```python
from build123d import *

# Parameters (mm, degrees)
F0_W     = 50.8
F0_H     = 50.8
F1_DEPTH = 25.4
F2_W     = 50.8
F2_H     = 25.4
F3_DEPTH = 25.4
F4_W     = 50.8
F4_H     = 76.2
F5_DEPTH = 25.4
F6_W     = 50.8
F6_H     = 101.6
F7_DEPTH = 25.4
F8_W     = 50.8
F8_H     = 127
F9_DEPTH = 25.4


with BuildPart() as f1:
    # F0 (on Top) → F1 (new body)
    with BuildSketch(Plane.XY):
        with Locations((25.4, 25.4)):
            Rectangle(F0_W, F0_H)
    extrude(amount=F1_DEPTH)

    # F2 (on face) → F3 (join)
    with BuildSketch(Plane.XY.offset(25.4)):
        with Locations((25.4, 38.1)):
            Rectangle(F2_W, F2_H)
    extrude(amount=F3_DEPTH)

    # F4 (on face) → F5 (join)
    with BuildSketch(Plane(origin=(0, 50.8, 0), x_dir=(-1, 0, 0), z_dir=(0, 1, 0))):
        with Locations((-25.4, 38.1)):
            Rectangle(F4_W, F4_H)
    extrude(amount=F5_DEPTH)

    # F6 (on face) → F7 (join)
    with BuildSketch(Plane(origin=(0, 0, 0), x_dir=(1, 0, 0), z_dir=(0, 0, -1))):
        with Locations((25.4, -25.4)):
            Rectangle(F6_W, F6_H)
    extrude(amount=F7_DEPTH)

    # F8 (on face) → F9 (join)
    with BuildSketch(Plane(origin=(0, 0, -25.4), x_dir=(1, 0, 0), z_dir=(0, 0, -1))):
        with Locations((25.4, -12.7)):
            Rectangle(F8_W, F8_H)
    extrude(amount=F9_DEPTH)


solid = f1.part
```
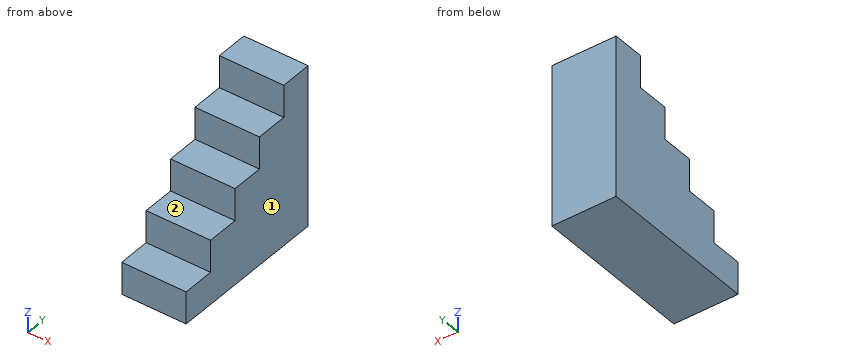
Verification items for the finished model (mm, model axes). Face numbers are marked on the shaded views. A direction names the side the tool comes from. Give positions to 0.01 mm unless a question says otherwise; leave off trailing zeros. Order: outer loops, then holes, each group sorted by start corner. A loop starts at its lowest first (then second) coordinate and runs counter-clockwise, first axis right, second up. Notation, with made-up numbers: M 55.5,62.25 L 84.5,62.25 A32 cw 84.5,96.25 Z; hole C 3,-28.75 d3. An arc over 180 degrees is marked long. Answer in a Markdown table with one row per item. Add a question column.
Item 1: Tool access check on the marked faces 1 and 2. Record the directions out of +Z, -Z, +X, -X, +Y, -Y that give a thin tool (end or side, any length) a straight path to the whole face; none if there is none.
Item 2: Gauge pin test, flat ends, axial feed: pin 1 (7.5 mm diameter, centred on x = 18, y = -13.5, fed in from +Z); pin 2 (12 mm diameter, centred on y = -27, z = -21, fed in from -X); pin 3 (7.5 mm diameter, centred on x = 18, z = 68.5, fed in from -Y); pin 4 (12 mm diameter, centred on x = 32, z = 31.5, fed in from -Y). Record the tip position at first contact, or that the pin passes through.
Item 3: Scan lines: probe 1 along Z at (x, y) = (36.5, -16); probe 2 along Z at (x, y) = (9, 19.5); probe 3 along Y at (x, z) = (14.5, -11). Record each from-to range of solid material in increasing order. Write a range as from..to.
Item 4: Section check A-A, the plane x = 30. Enter the section's corners in (y, z).
Item 5: Section check C-C, the plane y = 6. Enter the section's corners in (x, z), and give its area (3 significant figures).
Item 6: Section check B-B, the plane z = 30. Enter the section's corners in (x, y).
Filled sheet:
| question | item | result |
|---|---|---|
| 1 | face 1 | +Z, -Z, +X, +Y, -Y |
| 1 | face 2 | +Z, +X, -X, -Y |
| 2 | pin 1 | stops at z = 0 |
| 2 | pin 2 | stops at x = 0 |
| 2 | pin 3 | stops at y = 50.8 |
| 2 | pin 4 | stops at y = 25.4 |
| 3 | probe 1 | z = -50.8..0 |
| 3 | probe 2 | z = -50.8..25.4 |
| 3 | probe 3 | y = -25.4..76.2 |
| 4 | outline | M -50.8,-50.8 L 76.2,-50.8 L 76.2,76.2 L 50.8,76.2 L 50.8,50.8 L 25.4,50.8 L 25.4,25.4 L 0,25.4 L 0,0 L -25.4,0 L -25.4,-25.4 L -50.8,-25.4 Z |
| 5 | outline | M 0,-50.8 L 50.8,-50.8 L 50.8,25.4 L 0,25.4 Z |
| 5 | area | 3,870 mm^2 |
| 6 | outline | M 0,25.4 L 50.8,25.4 L 50.8,76.2 L 0,76.2 Z |
